Study the drawing (mm; zero at the part's minimum x, y, z) and answer. A direction names the side the tool comes from. Round coordinates to 2 decimals unless told otherwise and drop trailing zeros. Write each loop counter-clockwise with the first axis right and the second up, starting at its lowest first coordinate (ties: lowest second). Pieces come first, ordered by that corner, then holes. Notation, with made-up numbers: M 67.5,-35.5 L 104.5,-35.5 A30 cw 104.5,-7.5 Z; hole C 55.5,8 d11. An arc over 180 degrees is marked long. Write each question's results on one line, items separated by ' | '.
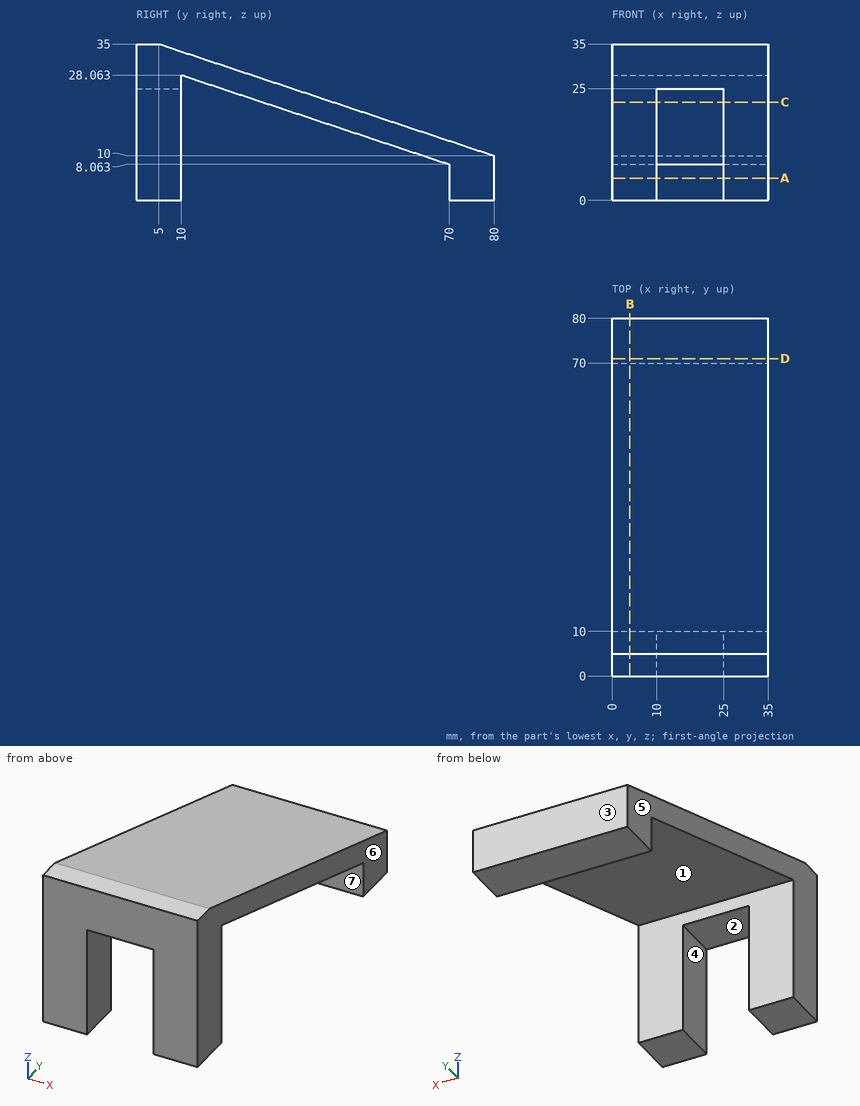
1) A tool of negligible diameter and unlimited length cuts with its end or side. For the marked faces 1, 2 and 3, from which of +Z, -Z, +X, -X, +Y, -Y can it reach the whole face along a straight path? Write none if from no direction.
Return value:
face 1: -Z, +X, -X | face 2: -Z, -Y | face 3: +Z, -Z, +X, -X, +Y
2) Section B-B (x = 4) is taken. Determine the outline of the cut face in (y, z), then the cut area to 3 significant figures.
Return value:
outline: M 0,0 L 10,0 L 10,28.06 L 70,8.06 L 70,0 L 80,0 L 80,10 L 5,35 L 0,35 Z | area: 779 mm²
3) Section C-C (z = 22) is taken. Determine the outline of the cut face in (x, y).
Return value:
outline: M 0,0 L 10,0 L 10,10 L 0,10 Z; M 0,28.19 L 35,28.19 L 35,44 L 0,44 Z; M 25,0 L 35,0 L 35,10 L 25,10 Z
4) Each of these flat-tipped pins is pushed along its axis until it touches: pin 1 (8 mm diameter, centred on x = 15, y = 6, fed in from -Z); pin 2 (2 mm diameter, centred on x = 12, y = 17, fed in from +Z); pin 3 (1.5 mm diameter, centred on x = 11.5, y = 18, fed in from +Z). Where does it stop, or does it pass through?
Return value:
pin 1: z = 25 | pin 2: z = 31.33 | pin 3: z = 30.92
5) The mould has two halves that part along X. Classify the marked faces 4, 5, 6 and 7: +X half, -X half, draft (parallel to the pull), parting line (faces both ways), or undercut.
Return value:
face 4: undercut | face 5: -X half | face 6: +X half | face 7: draft
6) Find the intervals of material crossed by line 1 (Y direction, x = 26.5, z = 3.5); line 2 (Z direction, x = 23.5, y = 58); line 3 (Z direction, x = 17.5, y = 11.5), in increasing order.
Return value:
line 1: 0 to 10, 70 to 80 | line 2: 12.06 to 17.33 | line 3: 27.56 to 32.83
7) Section A-A (z = 5) is taken. Determine the outline of the cut face in (x, y), then the cut area to 3 significant figures.
Return value:
outline: M 0,0 L 10,0 L 10,10 L 0,10 Z; M 0,70 L 35,70 L 35,80 L 0,80 Z; M 25,0 L 35,0 L 35,10 L 25,10 Z | area: 550 mm²
8) Section D-D (y = 71) is taken. Determine the outline of the cut face in (x, z).
Return value:
outline: M 0,0 L 35,0 L 35,13 L 0,13 Z
